Here's how the part is built. I have some questions about the finished solid (model axes, mm). A direction names the side the tool comes from. Coordinates: 2 decimals unless noted, no trailing zeros. Write each loop counter-clockwise with the first axis right and the second up, starting at its lowest first coordinate (ties: lowest second). Pieces come first, ordered by that corner, then holes. Notation, with made-up numbers: (-28, 22) - (30, 22) arc R26 cw to (30, 46) - close; hole circle Ø5 at (65.25, -7). An arc over 180 degrees is marked (long way). Answer in a Markdown table with one row per item. Add a question column.
Item 1: We'd pull the mould along X, two halves only. Please class faces 3 (the face through (83.986, 15.21, -69.297)), 4 (the face through (-53.986, 19.86, 39.297)), 5 (the face through (-1, 0, -1)): +X half, -X half, draft (parallel to the pull), parting line (faces both ways), or undercut.
Item 2: Imagine slicing it at D-D (y = 12.5). Please give me the cut outline in (x, z), plus the area to 3 significant figures.
Item 3: If I drill on probe 1 along X at (y, z) = (24.5, 55); probe 2 along Z at (x, y) = (70, 23); probe 3 along X at (y, z) = (19.75, 24), over which ranges is the centre line in solid material (lowest first)? Write a range as from..to.
Item 4: Imagine slicing it at C-C (x = -5). Please give me the cut outline in (y, z).
Item 5: Imagine slicing it at B-B (z = 0). Please give me the cut outline in (x, y).
Item 6: Which directions (+Z, -Z, +X, -X, +Y, -Y) give clear straight access to the entire face, cutting with the end or side of a thin tool? Please do faces 1 (the face through (83.986, 15.21, 69.297)), 2 (the face through (-1, 20, -45)).
Item 7: Imagine slicing it at A-A (y = 25.5). Please give me the cut outline in (x, z).
from build123d import *

# Parameters (mm, degrees)
SKETCH1_W                  = 180
SKETCH1_H                  = 150
BOSS_EXTRUDE1_DEPTH        = 30
F_16_0MM_DOWEL_HOLE1_D     = 16
F_16_0MM_DOWEL_HOLE1_DEPTH = 15
F_16_0MM_DOWEL_HOLE1_TIP   = 4.806884952
SKETCH5_W                  = 120
SKETCH5_H                  = 90
CUT_EXTRUDE1_DEPTH         = 20
FILLET1_R                  = 20
FILLET2_R                  = 20


with BuildPart() as part:
    # Sketch1 → Boss-Extrude1 (new body)
    with BuildSketch(Plane(origin=(0, 0, 0), x_dir=(1, 0, 0), z_dir=(0, 1, 0))):
        Rectangle(SKETCH1_W, SKETCH1_H)
    extrude(amount=BOSS_EXTRUDE1_DEPTH)

    # Ø16.0mm Dowel Hole1
    with Locations(Plane(origin=(-70, 30, 55), x_dir=(0, 0, 1), z_dir=(0, 1, 0))):
        with Locations((0, 0), (-110, 0), (-110, 140), (0, 140)):
            Hole(F_16_0MM_DOWEL_HOLE1_D / 2, depth=F_16_0MM_DOWEL_HOLE1_DEPTH)
            with Locations((0, 0, -(F_16_0MM_DOWEL_HOLE1_DEPTH + F_16_0MM_DOWEL_HOLE1_TIP / 2))):  # 118° drill point
                Cone(0, F_16_0MM_DOWEL_HOLE1_D / 2, F_16_0MM_DOWEL_HOLE1_TIP, mode=Mode.SUBTRACT)

    # Sketch5 → Cut-Extrude1 (cut)
    with BuildSketch(Plane(origin=(0, 30, 0), x_dir=(1, 0, 0), z_dir=(0, 1, 0))):
        Rectangle(SKETCH5_W, SKETCH5_H)
    extrude(amount=-CUT_EXTRUDE1_DEPTH, mode=Mode.SUBTRACT)

    # Fillet1
    fillet1_edges = [part.edges().sort_by_distance(p)[0] for p in [
        (60, 20, -45),
        (-60, 20, -45),
        (-60, 20, 45),
        (60, 20, 45),
    ]]
    fillet(fillet1_edges, radius=FILLET1_R)

    # Fillet2
    fillet2_edges = [part.edges().sort_by_distance(p)[0] for p in [
        (90, 15, 75),
        (90, 15, -75),
    ]]
    fillet(fillet2_edges, radius=FILLET2_R)


solid = part.part
Here are the results:
| question | item | result |
|---|---|---|
| 1 | face 3 | +X half |
| 1 | face 4 | undercut |
| 1 | face 5 | draft |
| 2 | outline | (-90, -75) - (70, -75) arc R20 ccw to (90, -55) - (90, 55) arc R20 ccw to (70, 75) - (-90, 75) - close; hole circle Ø7.68 at (-70, -55); hole circle Ø7.68 at (-70, 55); hole (-60, -25) arc R20 ccw to (-40, -45) - (40, -45) arc R20 ccw to (60, -25) - (60, 25) arc R20 ccw to (40, 45) - (-40, 45) arc R20 ccw to (-60, 25) - close; hole circle Ø7.68 at (70, -55); hole circle Ø7.68 at (70, 55) |
| 2 | area | 16,200 mm2 |
| 3 | probe 1 | x = -90..-78, -62..62, 78..90 |
| 3 | probe 2 | z = -75..-63, -47..47, 63..75 |
| 3 | probe 3 | x = -90..-60, 60..90 |
| 4 | outline | (0, -75) - (30, -75) - (30, -45) - (10, -45) - (10, 45) - (30, 45) - (30, 75) - (0, 75) - close |
| 5 | outline | (-90, 0) - (90, 0) - (90, 30) - (60, 30) - (60, 10) - (-60, 10) - (-60, 30) - (-90, 30) - close |
| 6 | face 1 | +Z, +X, +Y, -Y |
| 6 | face 2 | +Y |
| 7 | outline | (-90, -75) - (70, -75) arc R20 ccw to (90, -55) - (90, 55) arc R20 ccw to (70, 75) - (-90, 75) - close; hole circle Ø16 at (-70, -55); hole circle Ø16 at (-70, 55); hole (-60, -25) arc R20 ccw to (-40, -45) - (40, -45) arc R20 ccw to (60, -25) - (60, 25) arc R20 ccw to (40, 45) - (-40, 45) arc R20 ccw to (-60, 25) - close; hole circle Ø16 at (70, -55); hole circle Ø16 at (70, 55) |
